Could you check a few things on this model? Use its own coordinates, in mm. A direction names the side the tool comes from. Coordinates: 2 decimals unless noted, no trailing zeros. Loops run counter-clockwise (first coordinate to the right, second up) from the corner with the lowest first, then second, coordinate; pieces in that order, holes last. Notation, with made-up numbers: (46.5, 34) -> (105.5, 34) arc R29 ccw to (105.5, 58) -> close; hole circle Ø2 at (-0.5, 4.5). An arc over 180 degrees is marked (long way). One line per question, with ' | ' between items.
```python
from build123d import *

# Parameters (mm, degrees)
SKETCH1_W           = 119.48
SKETCH1_H           = 177.8
BOSS_EXTRUDE1_DEPTH = 5.13
CUT_EXTRUDE1_DEPTH  = 5.13
SKETCH5_W           = 5.13
SKETCH5_H           = 58.88
BOSS_EXTRUDE2_DEPTH = 5.13
SKETCH8_W           = 5.13
SKETCH8_H           = 58.88
BOSS_EXTRUDE3_DEPTH = 5.13


with BuildPart() as part:
    # Sketch1 → Boss-Extrude1 (new body)
    with BuildSketch(Plane(origin=(0, 0, 0), x_dir=(0, 0, -1), z_dir=(1, 0, 0))):
        with Locations((24.047197546, -50.943101868)):
            Rectangle(SKETCH1_W, SKETCH1_H)
    extrude(amount=BOSS_EXTRUDE1_DEPTH)

    # Sketch2 → Cut-Extrude1 (cut)
    with BuildSketch(Plane(origin=(5.13, 0, 0), x_dir=(0, 0, -1), z_dir=(1, 0, 0))):
        Polygon((-26.892802454, 37.956898132), (-23.895802454, 37.956898132), (-23.895802454, 33.961898132), (-22.536802454, 33.961898132), (-22.536802454, 31.794898132), (-23.895802454, 31.794898132), (-23.895802454, 25.587898132), (-26.892802454, 25.587898132), (-26.892802454, 31.794898132), (-28.251802454, 31.794898132), (-28.251802454, 33.961898132), (-26.892802454, 33.961898132), align=None)
        Polygon((71.987197546, 33.961898132), (71.987197546, 37.956898132), (74.984197546, 37.956898132), (74.984197546, 33.961898132), (76.343197546, 33.961898132), (76.343197546, 31.794898132), (74.984197546, 31.794898132), (74.984197546, 25.587898132), (71.987197546, 25.587898132), (71.987197546, 31.794898132), (70.628197546, 31.794898132), (70.628197546, 33.961898132), align=None)
        Polygon((76.343197546, -133.681101868), (74.984197546, -133.681101868), (74.984197546, -127.474101868), (71.987197546, -127.474101868), (71.987197546, -133.681101868), (70.628197546, -133.681101868), (70.628197546, -135.848101868), (71.987197546, -135.848101868), (71.987197546, -139.843101868), (74.984197546, -139.843101868), (74.984197546, -135.848101868), (76.343197546, -135.848101868), align=None)
        Polygon((-26.892802454, -139.843101868), (-23.895802454, -139.843101868), (-23.895802454, -135.848101868), (-22.536802454, -135.848101868), (-22.536802454, -133.681101868), (-23.895802454, -133.681101868), (-23.895802454, -127.474101868), (-26.892802454, -127.474101868), (-26.892802454, -133.681101868), (-28.251802454, -133.681101868), (-28.251802454, -135.848101868), (-26.892802454, -135.848101868), align=None)
    extrude(amount=-CUT_EXTRUDE1_DEPTH, mode=Mode.SUBTRACT)

    # Sketch5 → Boss-Extrude2 (add)
    with BuildSketch(Plane(origin=(0, 37.956898132, 0), x_dir=(1, 0, 0), z_dir=(0, 1, 0))):
        with Locations((2.565, 24.047197546)):
            Rectangle(SKETCH5_W, SKETCH5_H)
    extrude(amount=BOSS_EXTRUDE2_DEPTH)

    # Sketch8 → Boss-Extrude3 (add)
    with BuildSketch(Plane.XZ.offset(139.843101868)):
        with Locations((2.565, -24.047197546)):
            Rectangle(SKETCH8_W, SKETCH8_H)
    extrude(amount=BOSS_EXTRUDE3_DEPTH)


solid = part.part
```
Q1. For faces 1 (the face through (3, -138, -74.984)), 2 (the face through (3, -142, -53.487)), 3 (the face through (3, 37.957, 31)), which set-ups out of +Z, -Z, +X, -X, +Y, -Y let a thin tool reach every point of the face, with its end or its side?
Values follow:
face 1: +X, -X, -Y | face 2: -Z, +X, -X, -Y | face 3: +Z, +X, -X, +Y
Q2. Imagine slicing it at A-A on z = -59. Write out the boundary of the cut face in (x, y).
Values follow:
outline: (0, -139.84) -> (5.13, -139.84) -> (5.13, 37.96) -> (0, 37.96) -> close
Q3. For pin 1 (1 mm diameter, centred on x = 3.5, z = 19, fed in from -Y); pin 2 (1.1 mm diameter, centred on x = 2.5, z = 23.5, fed in from +Y); pin 3 (5 mm diameter, centred on y = -56, z = 8, fed in from -X), each with a flat end and sliding along its axis, tell me the tip position at first contact or that it passes through.
Values follow:
pin 1: stops at y = -139.84 | pin 2: stops at y = 37.96 | pin 3: stops at x = 0
Q4. We'd pull the mould along Z, two halves only. Please class faces 4 (the face through (3, -139.843, 15)), 5 (the face through (3, -52, 35.693)), 6 (the face through (3, -138, 26.893)): released by +Z, released by -Z, zero draft, split by the parting line, or undercut.
Values follow:
face 4: zero draft | face 5: released by +Z | face 6: undercut
Q5. Please list where these lines run through material, in increasing order: L1, parallel to Z at x = 0.5, y = 28; L2, parallel to Y at x = 2.7, z = 22. Write a range as [from, to].
Values follow:
L1: z = [-83.79, -74.98], [-71.99, 23.9], [26.89, 35.69] | L2: y = [-139.84, 37.96]
